from build123d import *

# Parameters (mm, degrees)
F0_R     = 10.4
F1_DEPTH = 26


with BuildPart() as f1:
    # F0 (on Top) → F1 (new body)
    with BuildSketch(Plane.XY):
        with Locations((-0.02051, -0.492754)):
            Circle(F0_R)
        with BuildLine():
            ThreePointArc((5.65055, 5.838841), (7.10127, 4.147317), (8.062501, 2.136875))
            ThreePointArc((8.062501, 2.136875), (8.334835, 1.068726), (8.466648, -0.025685))
            ThreePointArc((8.466648, -0.025685), (8.476279, -0.259131), (8.47949, -0.492754))
            ThreePointArc((8.47949, -0.492754), (8.245001, -2.475514), (7.55447, -4.348877))
            ThreePointArc((7.55447, -4.348877), (6.991744, -5.296742), (6.311085, -6.163813))
            ThreePointArc((6.311085, -6.163813), (4.619561, -7.614533), (2.609119, -8.575764))
            ThreePointArc((2.609119, -8.575764), (1.540969, -8.848098), (0.446559, -8.979911))
            ThreePointArc((0.446559, -8.979911), (-1.775343, -8.809638), (-3.876633, -8.067733))
            ThreePointArc((-3.876633, -8.067733), (-4.824498, -7.505007), (-5.691569, -6.824348))
            ThreePointArc((-5.691569, -6.824348), (-7.142289, -5.132824), (-8.10352, -3.122382))
            ThreePointArc((-8.10352, -3.122382), (-8.375854, -2.054233), (-8.507667, -0.959822))
            ThreePointArc((-8.507667, -0.959822), (-8.337394, 1.26208), (-7.595489, 3.36337))
            ThreePointArc((-7.595489, 3.36337), (-7.032763, 4.311235), (-6.352104, 5.178306))
            ThreePointArc((-6.352104, 5.178306), (-4.66058, 6.629026), (-2.650138, 7.590257))
            ThreePointArc((-2.650138, 7.590257), (-1.581989, 7.862591), (-0.487578, 7.994404))
            ThreePointArc((-0.487578, 7.994404), (1.734324, 7.82413), (3.835614, 7.082226))
            ThreePointArc((3.835614, 7.082226), (4.783479, 6.5195), (5.65055, 5.838841))
        make_face(mode=Mode.SUBTRACT)
        with BuildLine():
            ThreePointArc((-5.906331, -1.892612), (-6.069387, -0.609324), (-5.955895, 0.679294))
            Line((-5.955895, 0.679294), (-7.282285, 0.913172))
            ThreePointArc((-7.282285, 0.913172), (-7.448003, 0.868768), (-7.52051, 0.713278))
            Line((-7.52051, 0.713278), (-7.52051, -0.393065))
            ThreePointArc((-7.52051, -0.393065), (-7.5535, -0.50399), (-7.641748, -0.578857))
            Line((-7.641748, -0.578857), (-8.507667, -0.959822))
            ThreePointArc((-8.507667, -0.959822), (-8.375854, -2.054233), (-8.10352, -3.122382))
            Line((-8.10352, -3.122382), (-5.906331, -1.892612))
        make_face()
        with BuildLine():
            ThreePointArc((-5.172264, 2.679301), (-4.380139, 3.702021), (-3.388698, 4.532961))
            Line((-3.388698, 4.532961), (-4.16122, 5.636236))
            ThreePointArc((-4.16122, 5.636236), (-4.309799, 5.722019), (-4.471018, 5.66334))
            Line((-4.471018, 5.66334), (-5.25332, 4.881038))
            ThreePointArc((-5.25332, 4.881038), (-5.355083, 4.82593), (-5.470423, 4.835391))
            Line((-5.470423, 4.835391), (-6.352104, 5.178306))
            ThreePointArc((-6.352104, 5.178306), (-7.032763, 4.311235), (-7.595489, 3.36337))
            Line((-7.595489, 3.36337), (-5.172264, 2.679301))
        make_face()
        with BuildLine():
            ThreePointArc((-1.420368, 5.393068), (-0.13708, 5.556123), (1.151538, 5.442632))
            Line((1.151538, 5.442632), (1.385416, 6.769021))
            ThreePointArc((1.385416, 6.769021), (1.341012, 6.93474), (1.185522, 7.007246))
            Line((1.185522, 7.007246), (0.079179, 7.007246))
            ThreePointArc((0.079179, 7.007246), (-0.031746, 7.040237), (-0.106613, 7.128485))
            Line((-0.106613, 7.128485), (-0.487578, 7.994404))
            ThreePointArc((-0.487578, 7.994404), (-1.581989, 7.862591), (-2.650138, 7.590257))
            Line((-2.650138, 7.590257), (-1.420368, 5.393068))
        make_face()
        with BuildLine():
            ThreePointArc((3.151545, 4.659), (4.174265, 3.866876), (5.005205, 2.875435))
            Line((5.005205, 2.875435), (6.10848, 3.647957))
            ThreePointArc((6.10848, 3.647957), (6.194263, 3.796536), (6.135584, 3.957754))
            Line((6.135584, 3.957754), (5.353282, 4.740057))
            ThreePointArc((5.353282, 4.740057), (5.298174, 4.84182), (5.307635, 4.95716))
            Line((5.307635, 4.95716), (5.65055, 5.838841))
            ThreePointArc((5.65055, 5.838841), (4.783479, 6.5195), (3.835614, 7.082226))
            Line((3.835614, 7.082226), (3.151545, 4.659))
        make_face()
        with BuildLine():
            ThreePointArc((5.865312, 0.907105), (5.988306, 0.211973), (6.02949, -0.492754))
            ThreePointArc((6.02949, -0.492754), (6.000769, -1.081573), (5.914876, -1.664801))
            Line((5.914876, -1.664801), (7.241265, -1.89868))
            ThreePointArc((7.241265, -1.89868), (7.406984, -1.854275), (7.47949, -1.698785))
            Line((7.47949, -1.698785), (7.47949, -0.592443))
            ThreePointArc((7.47949, -0.592443), (7.512481, -0.481518), (7.600728, -0.40665))
            Line((7.600728, -0.40665), (8.466648, -0.025685))
            ThreePointArc((8.466648, -0.025685), (8.334835, 1.068726), (8.062501, 2.136875))
            Line((8.062501, 2.136875), (5.865312, 0.907105))
        make_face()
        with BuildLine():
            Line((7.55447, -4.348877), (5.131244, -3.664808))
            ThreePointArc((5.131244, -3.664808), (4.33912, -4.687528), (3.347679, -5.518468))
            Line((3.347679, -5.518468), (4.120201, -6.621744))
            ThreePointArc((4.120201, -6.621744), (4.26878, -6.707526), (4.429998, -6.648847))
            Line((4.429998, -6.648847), (5.2123, -5.866545))
            ThreePointArc((5.2123, -5.866545), (5.314064, -5.811437), (5.429404, -5.820899))
            Line((5.429404, -5.820899), (6.311085, -6.163813))
            ThreePointArc((6.311085, -6.163813), (6.991744, -5.296742), (7.55447, -4.348877))
        make_face()
        with BuildLine():
            Line((2.609119, -8.575764), (1.379349, -6.378575))
            ThreePointArc((1.379349, -6.378575), (0.096061, -6.54163), (-1.192557, -6.428139))
            Line((-1.192557, -6.428139), (-1.426436, -7.754529))
            ThreePointArc((-1.426436, -7.754529), (-1.382031, -7.920247), (-1.226541, -7.992754))
            Line((-1.226541, -7.992754), (-0.120199, -7.992754))
            ThreePointArc((-0.120199, -7.992754), (-0.009274, -8.025744), (0.065594, -8.113992))
            Line((0.065594, -8.113992), (0.446559, -8.979911))
            ThreePointArc((0.446559, -8.979911), (1.540969, -8.848098), (2.609119, -8.575764))
        make_face()
        with BuildLine():
            Line((-3.876633, -8.067733), (-3.192564, -5.644508))
            ThreePointArc((-3.192564, -5.644508), (-4.215284, -4.852383), (-5.046224, -3.860942))
            Line((-5.046224, -3.860942), (-6.1495, -4.633464))
            ThreePointArc((-6.1495, -4.633464), (-6.235282, -4.782043), (-6.176604, -4.943262))
            Line((-6.176604, -4.943262), (-5.394301, -5.725564))
            ThreePointArc((-5.394301, -5.725564), (-5.339193, -5.827327), (-5.348655, -5.942667))
            Line((-5.348655, -5.942667), (-5.691569, -6.824348))
            ThreePointArc((-5.691569, -6.824348), (-4.824498, -7.505007), (-3.876633, -8.067733))
        make_face()
    extrude(amount=F1_DEPTH)


solid = f1.part
Can you work these out from the model? Positions are in its coordinate system, mm. Give positions to 0.01 mm unless a question says otherwise; leave off trailing zeros. Loops run counter-clockwise (first coordinate to the right, second up) from the corner with the lowest first, then second, coordinate; pieces in that order, holes last. Notation, with made-up numbers: M 86,10 L 139,10 A18 ccw 139,24 Z; hole C 62.5,54.5 d3. An arc over 180 degrees is marked long. One line per item, written item: value.
1) Imagine slicing it at A-A on y = -2.25. Write out the boundary of the cut face in (x, z), and give its area (3 significant figures).
Geometry check:
outline: M -10.27,0 L -6.54,0 L -6.54,26 L -10.27,26 Z; M 8.3,0 L 10.23,0 L 10.23,26 L 8.3,26 Z
area: 147 mm²
2) Please list where these lines run through material, in increasing order: line 1 (X direction, y = 4.25, z = 7.25); line 2 (Y direction, x = -0.25, z = 14.5); line 3 (Y direction, x = -5, z = 18.25).
Geometry check:
line 1: x = -9.28 to -3.78, 3.74 to 5.84, 7.03 to 9.24
line 2: y = -10.89 to -8.99, -7.99 to -6.54, 5.55 to 7.45, 8 to 9.9
line 3: y = -9.62 to -3.93, 2.94 to 5.13, 6.4 to 8.64
3) Thinking about a two-plate mould opening in Y: for faces 1 (the face through (4.5, -5, 0)), 2 (the face through (-1.308, -7.082, 12.818)), which applies, +Y half, -Y half, draft (parallel to the pull), parting line (faces both ways), or undercut?
Geometry check:
face 1: draft
face 2: undercut
4) I'm going to push flat-ended pins straight in: pin 1 (1.2 mm diameter, centred on y = -1.5, z = 7, fed in from +X); pin 2 (1 mm diameter, centred on x = 1, z = 10.5, fed in from -Y); pin 3 (4 mm diameter, centred on y = 4.5, z = 22.5, fed in from +X). Where does each tip first touch, or does it pass through?
Geometry check:
pin 1: stops at x = 10.37
pin 2: stops at y = -10.88
pin 3: stops at x = 9.94
